```python
from build123d import *

# Parameters (mm, degrees)
F1_DEPTH = 6.35


with BuildPart() as f1:
    # F0 (on Front) → F1 (new body)
    with BuildSketch(Plane.XZ):
        with BuildLine():
            Line((0, 11.43), (0, 12.7))
            ThreePointArc((0, 12.7), (-0.996431, 12.66085), (-1.986718, 12.543642))
            Line((-1.986718, 12.543642), (-1.788046, 11.289278))
            ThreePointArc((-1.788046, 11.289278), (-2.668281, 11.114188), (-3.532064, 10.870576))
            Line((-3.532064, 10.870576), (-3.924516, 12.078418))
            ThreePointArc((-3.924516, 12.078418), (-4.500251, 12.385881), (-5.151037, 12.435703))
            ThreePointArc((-5.151037, 12.435703), (-5.575982, 11.940298), (-5.765679, 11.315783))
            Line((-5.765679, 11.315783), (-5.189111, 10.184205))
            ThreePointArc((-5.189111, 10.184205), (-5.972159, 9.745677), (-6.718385, 9.247064))
            Line((-6.718385, 9.247064), (-7.464873, 10.274516))
            ThreePointArc((-7.464873, 10.274516), (-8.107441, 10.389019), (-8.741771, 10.235298))
            ThreePointArc((-8.741771, 10.235298), (-8.992829, 9.632825), (-8.980256, 8.980256))
            Line((-8.980256, 8.980256), (-8.082231, 8.082231))
            ThreePointArc((-8.082231, 8.082231), (-8.69144, 7.423191), (-9.247064, 6.718385))
            Line((-9.247064, 6.718385), (-10.274516, 7.464873))
            ThreePointArc((-10.274516, 7.464873), (-10.921018, 7.375207), (-11.476799, 7.032992))
            ThreePointArc((-11.476799, 7.032992), (-11.529396, 6.382424), (-11.315783, 5.765679))
            Line((-11.315783, 5.765679), (-10.184205, 5.189111))
            ThreePointArc((-10.184205, 5.189111), (-10.559943, 4.374072), (-10.870576, 3.532064))
            Line((-10.870576, 3.532064), (-12.078418, 3.924516))
            ThreePointArc((-12.078418, 3.924516), (-12.665569, 3.639458), (-13.088399, 3.142246))
            ThreePointArc((-13.088399, 3.142246), (-12.937384, 2.507267), (-12.543642, 1.986718))
            Line((-12.543642, 1.986718), (-11.289278, 1.788046))
            ThreePointArc((-11.289278, 1.788046), (-11.394765, 0.896787), (-11.43, 0))
            Line((-11.43, 0), (-12.7, 0))
            ThreePointArc((-12.7, 0), (-13.170327, -0.452545), (-13.418814, -1.056084))
            ThreePointArc((-13.418814, -1.056084), (-13.078972, -1.613319), (-12.543642, -1.986718))
            Line((-12.543642, -1.986718), (-11.289278, -1.788046))
            ThreePointArc((-11.289278, -1.788046), (-11.114188, -2.668281), (-10.870576, -3.532064))
            Line((-10.870576, -3.532064), (-12.078418, -3.924516))
            ThreePointArc((-12.078418, -3.924516), (-12.385881, -4.500251), (-12.435703, -5.151037))
            ThreePointArc((-12.435703, -5.151037), (-11.940298, -5.575982), (-11.315783, -5.765679))
            Line((-11.315783, -5.765679), (-10.184205, -5.189111))
            ThreePointArc((-10.184205, -5.189111), (-9.745677, -5.972159), (-9.247064, -6.718385))
            Line((-9.247064, -6.718385), (-10.274516, -7.464873))
            ThreePointArc((-10.274516, -7.464873), (-10.389019, -8.107441), (-10.235298, -8.741771))
            ThreePointArc((-10.235298, -8.741771), (-9.632825, -8.992829), (-8.980256, -8.980256))
            Line((-8.980256, -8.980256), (-8.082231, -8.082231))
            ThreePointArc((-8.082231, -8.082231), (-7.423191, -8.69144), (-6.718385, -9.247064))
            Line((-6.718385, -9.247064), (-7.464873, -10.274516))
            ThreePointArc((-7.464873, -10.274516), (-7.375207, -10.921018), (-7.032992, -11.476799))
            ThreePointArc((-7.032992, -11.476799), (-6.382424, -11.529396), (-5.765679, -11.315783))
            Line((-5.765679, -11.315783), (-5.189111, -10.184205))
            ThreePointArc((-5.189111, -10.184205), (-4.374072, -10.559943), (-3.532064, -10.870576))
            Line((-3.532064, -10.870576), (-3.924516, -12.078418))
            ThreePointArc((-3.924516, -12.078418), (-3.639458, -12.665569), (-3.142246, -13.088399))
            ThreePointArc((-3.142246, -13.088399), (-2.507267, -12.937384), (-1.986718, -12.543642))
            Line((-1.986718, -12.543642), (-1.788046, -11.289278))
            ThreePointArc((-1.788046, -11.289278), (-0.896787, -11.394765), (0, -11.43))
            Line((0, -11.43), (0, -12.7))
            ThreePointArc((0, -12.7), (0.452545, -13.170327), (1.056084, -13.418814))
            ThreePointArc((1.056084, -13.418814), (1.613319, -13.078972), (1.986718, -12.543642))
            Line((1.986718, -12.543642), (1.788046, -11.289278))
            ThreePointArc((1.788046, -11.289278), (2.668281, -11.114188), (3.532064, -10.870576))
            Line((3.532064, -10.870576), (3.924516, -12.078418))
            ThreePointArc((3.924516, -12.078418), (4.500251, -12.385881), (5.151037, -12.435703))
            ThreePointArc((5.151037, -12.435703), (5.575982, -11.940298), (5.765679, -11.315783))
            Line((5.765679, -11.315783), (5.189111, -10.184205))
            ThreePointArc((5.189111, -10.184205), (5.972159, -9.745677), (6.718385, -9.247064))
            Line((6.718385, -9.247064), (7.464873, -10.274516))
            ThreePointArc((7.464873, -10.274516), (8.107441, -10.389019), (8.741771, -10.235298))
            ThreePointArc((8.741771, -10.235298), (8.992829, -9.632825), (8.980256, -8.980256))
            Line((8.980256, -8.980256), (8.082231, -8.082231))
            ThreePointArc((8.082231, -8.082231), (8.69144, -7.423191), (9.247064, -6.718385))
            Line((9.247064, -6.718385), (10.274516, -7.464873))
            ThreePointArc((10.274516, -7.464873), (10.921018, -7.375207), (11.476799, -7.032992))
            ThreePointArc((11.476799, -7.032992), (11.529396, -6.382424), (11.315783, -5.765679))
            Line((11.315783, -5.765679), (10.184205, -5.189111))
            ThreePointArc((10.184205, -5.189111), (10.559943, -4.374072), (10.870576, -3.532064))
            Line((10.870576, -3.532064), (12.078418, -3.924516))
            ThreePointArc((12.078418, -3.924516), (12.665569, -3.639458), (13.088399, -3.142246))
            ThreePointArc((13.088399, -3.142246), (12.937384, -2.507267), (12.543642, -1.986718))
            Line((12.543642, -1.986718), (11.289278, -1.788046))
            ThreePointArc((11.289278, -1.788046), (11.394765, -0.896787), (11.43, 0))
            Line((11.43, 0), (12.7, 0))
            ThreePointArc((12.7, 0), (13.170327, 0.452545), (13.418814, 1.056084))
            ThreePointArc((13.418814, 1.056084), (13.078972, 1.613319), (12.543642, 1.986718))
            Line((12.543642, 1.986718), (11.289278, 1.788046))
            ThreePointArc((11.289278, 1.788046), (11.114188, 2.668281), (10.870576, 3.532064))
            Line((10.870576, 3.532064), (12.078418, 3.924516))
            ThreePointArc((12.078418, 3.924516), (12.385881, 4.500251), (12.435703, 5.151037))
            ThreePointArc((12.435703, 5.151037), (11.940298, 5.575982), (11.315783, 5.765679))
            Line((11.315783, 5.765679), (10.184205, 5.189111))
            ThreePointArc((10.184205, 5.189111), (9.745677, 5.972159), (9.247064, 6.718385))
            Line((9.247064, 6.718385), (10.274516, 7.464873))
            ThreePointArc((10.274516, 7.464873), (10.389019, 8.107441), (10.235298, 8.741771))
            ThreePointArc((10.235298, 8.741771), (9.632825, 8.992829), (8.980256, 8.980256))
            Line((8.980256, 8.980256), (8.082231, 8.082231))
            ThreePointArc((8.082231, 8.082231), (7.423191, 8.69144), (6.718385, 9.247064))
            Line((6.718385, 9.247064), (7.464873, 10.274516))
            ThreePointArc((7.464873, 10.274516), (7.375207, 10.921018), (7.032992, 11.476799))
            ThreePointArc((7.032992, 11.476799), (6.382424, 11.529396), (5.765679, 11.315783))
            Line((5.765679, 11.315783), (5.189111, 10.184205))
            ThreePointArc((5.189111, 10.184205), (4.374072, 10.559943), (3.532064, 10.870576))
            Line((3.532064, 10.870576), (3.924516, 12.078418))
            ThreePointArc((3.924516, 12.078418), (3.639458, 12.665569), (3.142246, 13.088399))
            ThreePointArc((3.142246, 13.088399), (2.507267, 12.937384), (1.986718, 12.543642))
            Line((1.986718, 12.543642), (1.788046, 11.289278))
            ThreePointArc((1.788046, 11.289278), (0.896787, 11.394765), (0, 11.43))
        make_face()
        with BuildLine():
            ThreePointArc((-1.986718, 12.543642), (-0.996431, 12.66085), (0, 12.7))
            ThreePointArc((0, 12.7), (-0.452545, 13.170327), (-1.056084, 13.418814))
            ThreePointArc((-1.056084, 13.418814), (-1.613319, 13.078972), (-1.986718, 12.543642))
        make_face()
    extrude(amount=F1_DEPTH)


solid = f1.part
```
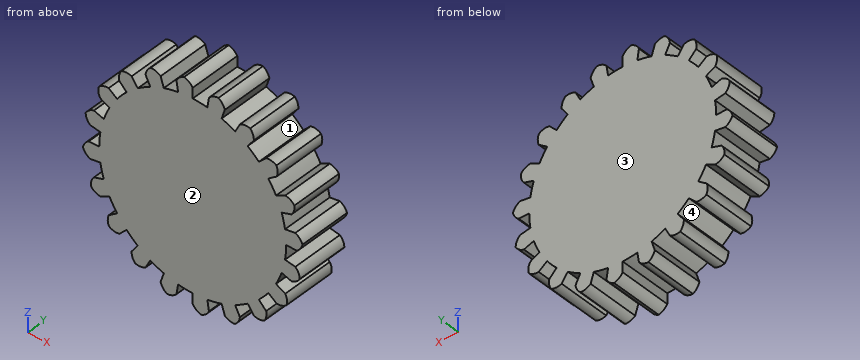
Could you check a few things on this model? Use its own coordinates, in mm. Face numbers are marked on the shaded views. A direction names the side the tool comes from. Round coordinates to 2 decimals unless told otherwise and drop trailing zeros. Loops run counter-clockwise (first coordinate to the right, second up) from the corner with the lowest first, then second, coordinate; pieces in that order, holes last. Notation, with made-up numbers: (-36, 37.25) -> (16, 37.25) arc R21 cw to (16, 74.25) -> close; hole circle Ø11 at (33.25, 55). An arc over 180 degrees is marked (long way). One line per question, with ' | ' between items.
(1) If I drill on probe 1 along Z at (x, y) = (-10.25, -5.5); probe 2 along X at (y, z) = (-4, 7); probe 3 along X at (y, z) = (-3.75, 9.5), over which ranges is the centre line in solid material (lowest first)?
Model answer:
probe 1: z = -8.71 to -7.45, -5.22 to 5.06, 5.22 to 7.45 | probe 2: x = -11.49 to -9.63, -9.04 to 9.63 | probe 3: x = -9.01 to -6.9, -6.36 to 6.9
(2) If we section it at A-A on z = -6.25: List the corners of the cut face in (x, y) for me, and give its area (3 significant figures).
Model answer:
outline: (-9.57, -6.35) -> (11.51, -6.35) -> (11.51, 0) -> (-9.57, 0) -> close | area: 134 mm^2
(3) For pin 1 Ø1 at (x, y) = (8, -5) entering from -Z; pin 2 Ø0.6 at (x, y) = (-12.5, -2) entering from +Z; pin 3 Ø0.6 at (y, z) = (-3, -12) entering from -X, each with a flat end and sliding along its axis, tell me the tip position at first contact or that it passes through.
Model answer:
pin 1: stops at z = -10.39 | pin 2: stops at z = 3.89 | pin 3: stops at x = -3.92
(4) Thinking about a two-plate mould opening in Z: for the marked faces 3 and 4, which applies, released by +Z, released by -Z, zero draft, split by the parting line, or undercut?
Model answer:
face 3: zero draft | face 4: undercut
(5) For the marked faces 1 and 2, which set-ups out of +Z, -Z, +X, -X, +Y, -Y let a thin tool reach every point of the face, with its end or its side?
Model answer:
face 1: +Y, -Y | face 2: +Z, -Z, +X, -X, -Y
